Read the model definition and answer for the solid it produces. Units are mm, in the model's axes. Face numbers are marked on the shaded views. Round coordinates to 2 decimals unless told otherwise and drop trailing zeros. Order: outer loops, then holes, each group sorted by start corner. A loop starts at its lowest first (then second) coordinate and runs counter-clockwise, first axis right, second up.
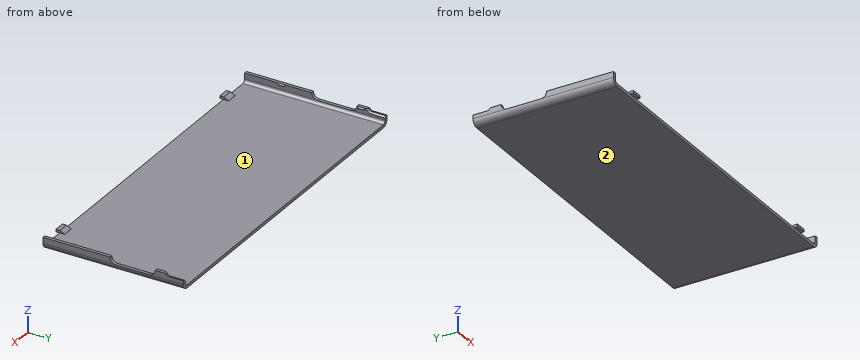
Autodesk Inventor part; units mm, degrees
ref_plane "Work Plane1" through (0, 13.97, 0) normal (0, 1, 0) x (-1, 0, 0)
ref_plane "Work Plane2" through (0, 16.51, 0) normal (0, 1, 0) x (-1, 0, 0)
ref_plane "Work Plane3" through (0, 46.99, 0) normal (0, 1, 0) x (-1, 0, 0)
sketch "Sketch1" plane through (0, 0, 0) normal (0, 1, 0) x (-1, 0, 0)
  line L0 (-70.1675, 4.953) -> (70.1675, 4.953) construction
  line L1 (70.1675, 4.953) -> (70.1675, 0) construction
  line L2 (70.1675, 0) -> (-70.1675, 0) construction
  line L3 (-70.1675, 0) -> (-70.1675, 4.953) construction
  line L4 (-67.6275, 0) -> (67.6275, 0)
  arc A0 (67.6275, 0) -> (70.1675, 2.54) centre (67.6275, 2.54) ccw
  line L5 (70.1675, 2.54) -> (70.1675, 4.953)
  arc A1 (-70.1675, 2.54) -> (-67.6275, 0) centre (-67.6275, 2.54) ccw
  line L6 (-70.1675, 2.54) -> (-70.1675, 4.953)
  line L7 (-68.8975, 4.953) -> (-68.8975, 2.54)
  arc A2 (-68.8975, 2.54) -> (-67.6275, 1.27) centre (-67.6275, 2.54) ccw
  line L8 (-67.6275, 1.27) -> (67.6275, 1.27)
  arc A3 (67.6275, 1.27) -> (68.8975, 2.54) centre (67.6275, 2.54) ccw
  line L9 (68.8975, 2.54) -> (68.8975, 4.953)
  line L10 (-70.1675, 4.953) -> (-68.8975, 4.953)
  line L11 (68.8975, 4.953) -> (70.1675, 4.953)
  point P0 (0, 0)
  point P1 (0, 0)
  dimension "d0" = 140.335
  dimension "d1" = 4.953
  dimension "d2" = 1.27
  dimension "d3" = 1.27
extrude "Extrusion1" add sketch "Sketch1" along normal blind 58.166
sketch "Sketch2" plane through (-67.6275, 0, 1.27) normal (0, 0, 1) x (1, 0, 0)
  line L0 (-2.54, 0) -> (-2.54, 58.166)
  line L1 (137.795, 0) -> (137.795, 58.166)
  line L2 (0, 0) -> (135.255, 0)
  line L3 (8.89, 2.159) -> (13.3858, 2.159)
  line L4 (13.3858, 2.159) -> (13.3858, -1.524)
  line L5 (13.3858, -1.524) -> (8.89, -1.524)
  line L6 (8.89, -1.524) -> (8.89, 2.159)
  point P0 (67.6275, 0)
  dimension "d6" = 4.4958
  dimension "d7" = 11.43
  dimension "d8" = 3.683
  dimension "d9" = 1.524
extrude "Extrusion2" add sketch "Sketch2" along normal blind 1.016
chamfer "Chamfer2" distance 2.032 distance2 1.016 1 edges at (-56.4896, 2.159, 2.286) measured on face at (-57.2389, 0.9313, 2.286)
sketch "Sketch3" plane through (0, 0, 0) normal (1, 0, 0) x (0, 1, 0)
  line L0 (0, 4.953) -> (58.166, 4.953)
  line L1 (0, 2.54) -> (0, 4.953)
  line L2 (58.166, 2.54) -> (58.166, 4.953)
  line L3 (0, 0) -> (58.166, 0)
  line L4 (0, 0) -> (58.166, 0)
  line L5 (46.474, 4.953) -> (27.694, 4.953) construction
  line L6 (44.0182, 2.4972) -> (30.1498, 2.4972)
  line L7 (30.1498, 7.4088) -> (44.0182, 7.4088)
  arc A0 (44.0182, 2.4972) -> (44.0182, 7.4088) centre (44.0182, 4.953) ccw
  arc A1 (30.1498, 7.4088) -> (30.1498, 2.4972) centre (30.1498, 4.953) ccw
  line L8 (58.166, 4.0386) -> (52.3421, 4.0386)
  line L9 (51.444, 4.4106) -> (50.9016, 4.953)
  arc A2 (51.444, 4.4106) -> (52.3421, 4.0386) centre (52.3421, 5.3086) ccw
  point P0 (0, 0)
  point P1 (37.084, 4.953)
  point P2 (51.816, 4.0386)
  dimension "d12" = 18.78
  dimension "d13" = 2.4558
  dimension "d15" = 2.4972
  dimension "d16" = 135
  dimension "d17" = 6.35
  dimension "d18" = 0.9144
  dimension "d19" = 1.27
  dimension "d36" = 37.084
extrude "Extrusion3" cut sketch "Sketch3" along normal through all both and the other way through all
chamfer "Chamfer1" distance 0.635 angle 45 6 edges at (-68.8975, 55.254, 4.0386) (-68.8975, 51.856, 4.1353) (-68.8975, 51.1728, 4.6818) (68.8975, 55.254, 4.0386) (68.8975, 51.856, 4.1353) (68.8975, 51.1728, 4.6818)
ref_plane "Work Plane1" through (0, 13.97, 0) normal (0, 1, 0) x (-1, 0, 0)
ref_plane "Work Plane2" through (0, 16.51, 0) normal (0, 1, 0) x (-1, 0, 0)
ref_plane "Work Plane3" through (0, 46.99, 0) normal (0, 1, 0) x (-1, 0, 0)
ref_plane "Work Plane4" through (0, 49.53, 0) normal (0, 1, 0) x (-1, 0, 0)
sketch "Sketch6" plane through (0, 0, 0) normal (0, 1, 0) x (-1, 0, 0)
  line L0 (-68.8975, 2.54) -> (-68.8975, 4.953)
  arc A0 (-68.8975, 2.54) -> (-67.6275, 1.27) centre (-67.6275, 2.54) ccw
  line L1 (-68.8975, 4.953) -> (-68.3895, 4.5009)
  line L2 (-68.3895, 4.5009) -> (-68.8975, 4.0488)
  line L3 (-68.3895, 4.5009) -> (-68.8975, 4.5009) construction
  point P0 (0, 0)
  dimension "d25" = 3.683
  dimension "d26" = 2.7788
  dimension "d27" = 0.508
extrude "Extrusion4" add sketch "Sketch6" along normal up to surface (2.54 mm away) from surface at 13.97
extrude "Extrusion5" add sketch "Sketch6" along normal up to surface (2.54 mm away) from surface at 46.99
mirror "Mirror1" about plane through (0, 0, 0) normal (1, 0, 0) of "Extrusion2", "Extrusion4", "Extrusion5", "Chamfer2"
properties part number "KTR-009"
Q1. A cutting plane is placed at C-C, the plane y = 54.5. Give the vertices of the cut face in (x, z), plus the area to 3 significant figures.
Outcome:
outline: (-70.17, 2.54) arc R2.54 ccw to (-67.63, 0) - (67.63, 0) arc R2.54 ccw to (70.17, 2.54) - (70.17, 4.04) - (69.53, 4.04) - (68.9, 3.4) - (68.9, 2.54) arc R1.27 cw to (67.63, 1.27) - (-67.63, 1.27) arc R1.27 cw to (-68.9, 2.54) - (-68.9, 3.4) - (-69.53, 4.04) - (-70.17, 4.04) - close
area: 183 mm2
Q2. For a pull along X with two mould halves and no side action, classify the marked faces 1 and 2 as released by +X, released by -X, zero draft, split by the parting line, or undercut.
Outcome:
face 1: undercut
face 2: zero draft
Q3. Straight lines are drawn through the part: probe 1 along X at (y, z) = (20, 3.05); probe 2 along Y at (x, z) = (-12.5, 0.75); probe 3 along Z at (x, y) = (9.5, 46.5). For each, find the intervals that lie inside material, in ascending order.
Outcome:
probe 1: x = -70.17 to -68.9, 68.9 to 70.17
probe 2: y = 0 to 58.17
probe 3: z = 0 to 1.27
Q4. Flat-ended cylindrical pins translate along their axes: pin 1 (1.3 mm diameter, centred on x = 57.5, y = -1, fed in from +Z); pin 2 (0.6 mm diameter, centred on x = -68.5, z = 4.5, fed in from -Y); pin 3 (1.4 mm diameter, centred on x = 69.5, y = 38, fed in from +Z). Find the tip coordinate at first contact, or state that the pin passes through.
Outcome:
pin 1: stops at z = 2.29
pin 2: stops at y = 13.97
pin 3: stops at z = 2.5
Q5. A cutting plane is placed at A-A, the plane y = 10. Give the vertices of the cut face in (x, z).
Outcome:
outline: (-70.17, 2.54) arc R2.54 ccw to (-67.63, 0) - (67.63, 0) arc R2.54 ccw to (70.17, 2.54) - (70.17, 4.95) - (68.9, 4.95) - (68.9, 2.54) arc R1.27 cw to (67.63, 1.27) - (-67.63, 1.27) arc R1.27 cw to (-68.9, 2.54) - (-68.9, 4.95) - (-70.17, 4.95) - close
Q6. A cutting plane is placed at B-B, the plane x = 23.5. Give the vertices of the cut face in (y, z).
Outcome:
outline: (0, 0) - (58.17, 0) - (58.17, 1.27) - (0, 1.27) - close
